Could you check a few things on this model? Use its own coordinates, in mm. A direction names the side the tool comes from. Give positions to 0.01 mm unless a question says otherwise; leave off trailing zeros. Order: outer loops, then holes, each group sorted by start corner. A loop starts at its lowest first (then second) coordinate and runs counter-clockwise, first axis right, second up. Notation, with made-up numbers: M 10,74.5 L 62,74.5 A11 cw 62,85.5 Z; hole C 70.5,-25 d9. An arc over 180 degrees is marked long. Answer in a Markdown table with one row per item. Add a question column.
```python
from build123d import *

# Parameters (mm, degrees)
BASEHEAD_DEPTH = 6.4
HEADFILLET_R   = 0.4
SKETCH4_W      = 0.6
SKETCH4_H      = 11.237604307


with BuildPart() as part:
    # Sketch1 → BaseHead (new body)
    with BuildSketch(Plane(origin=(0, 0, 0), x_dir=(0, 0, -1), z_dir=(1, 0, 0))):
        Polygon((8, 4.618802154), (8, -4.618802154), (0, -9.237604307), (-8, -4.618802154), (-8, 4.618802154), (0, 9.237604307), align=None)
    extrude(amount=BASEHEAD_DEPTH)

    # BodySke → BaseBody (revolve)
    with BuildSketch(Plane.XY):
        Polygon((0, 0), (66.4, 0), (66.4, 4.172), (65.572, 5), (0, 5), align=None)
    revolve(axis=Axis((0, 0, 0), (1, 0, 0)))

    # HeadFillet
    headfillet_edges = [part.edges().sort_by_distance(p)[0] for p in [
        (6.4, -5, 0),
    ]]
    fillet(headfillet_edges, radius=HEADFILLET_R)

    # Sketch3 → HeadChamfer (revolve, cut)
    with BuildSketch(Plane.XY):
        Polygon((0, 8), (3.601282526, 14.237604307), (3.601282526, 19.237604307), (-10, 19.237604307), (-10, 8), align=None)
    revolve(axis=Axis((0, 0, 0), (1, 0, 0)), mode=Mode.SUBTRACT)

    # Sketch4 → BearingFace (revolve, cut)
    with BuildSketch(Plane.XY):
        with Locations((6.1, 13.618802154)):
            Rectangle(SKETCH4_W, SKETCH4_H)
    revolve(axis=Axis((0, 0, 0), (1, 0, 0)), mode=Mode.SUBTRACT)


solid = part.part
```
1. For faces 1 (the flat face through (5.8, 4, 7.2)), 2 (the cylindrical face through (6.104, -6.349, -4.868)), 3 (the flat face through (5.8, -8.3, 0)), 4 (the flat face through (5.8, -4.2, 7.2)), which set-ups out of +Z, -Z, +X, -X, +Y, -Y let a thin tool reach every point of the face, with its end or its side?
2. If I drill on line 1 along Y through (x, z) = (8, 3); line 2 along Y through (x, z) = (6, -0.25); line 3 along X through (y, z) = (-4.5, -3.75), over which ranges is the centre line in solid material (lowest first)? Write a range as [from, to].
3. Suppose I cut it at A-A on x = 16. List the corners of the cut face in (y, z) for me, plus the area to 3 significant figures.
4. Will these pins go through, and if not, where does the flat tip stop? P1, Ø1.8, axis at y = 7.5, z = 1, coming from the +X side; P2, Ø4, axis at x = 8.5, z = 6, coming from the -Y side; P3, Ø1.5, axis at x = 41.5, z = 5, coming from the -Y side.
Findings below:
| question | item | result |
|---|---|---|
| 1 | face 1 | +Z, +X, +Y |
| 1 | face 2 | +X |
| 1 | face 3 | +X, -Y |
| 1 | face 4 | +Z, +X, -Y |
| 2 | line 1 | [-4, 4] |
| 2 | line 2 | [-8, 8] |
| 2 | line 3 | [0, 6.4] |
| 3 | outline | C 0,0 d10 |
| 3 | area | 78.5 mm2 |
| 4 | P1 | x = 6.4 |
| 4 | P2 | y = -3 |
| 4 | P3 | y = -2.63 |
